Answer from the drawing. Dimensions are ordinates in mm from the lowest x, y and z of the part. A direction names the side the tool comes from. Round coordinates to 2 decimals unless told otherwise and drop trailing zeros. Write each loop counter-clockwise with the first axis right and the second up, starting at its lowest first coordinate (ties: lowest second). Pieces come first, ordered by that corner, then holes.
1. Find section A-A (y = 14.92). Write down the section's boundary in (x, z).
2. Flat-ended cylindrical pins translate along their axes: pin 1 Ø5 at (y, z) = (11.5, 9) entering from -X; pin 2 Ø1.5 at (x, z) = (1, 1.5) entering from -Y; pin 3 Ø1.5 at (x, z) = (1, 1) entering from +Y; pin 4 Ø1.5 at (x, y) = (1, 12.5) entering from -Z. Find the tip coordinate at first contact, or state that the pin passes through.
3. A tool of negligible diameter and unlimited length cuts with its end or side. For the marked faces 5, 6, 7, 8 and 9, from which of +Z, -Z, +X, -X, +Y, -Y can it reach the whole face along a straight path? Write none if from no direction.
4. Find section C-C (x = 0.75). Write down the section's boundary in (y, z), and give its area (3 significant figures).
5. Find section B-B (z = 5.91). Write down the section's boundary in (x, y).
6. Find section D-D (z = 1.5). Write down the section's boundary in (x, y).
7. Straight lines are drawn through the part: probe 1 along Y at (x, z) = (1.9, 5.91); probe 2 along Z at (x, y) = (0.6, 5); probe 3 along Y at (x, z) = (1.95, 7). For each, find the intervals that lie inside material, in ascending order.
8. Determine the mould class of the marked faces 1, 2, 3 and 4 for opening direction Z: pulls with the +Z half, pulls with the -Z half, needs draft (parallel to the pull), parting line crosses it, or undercut.
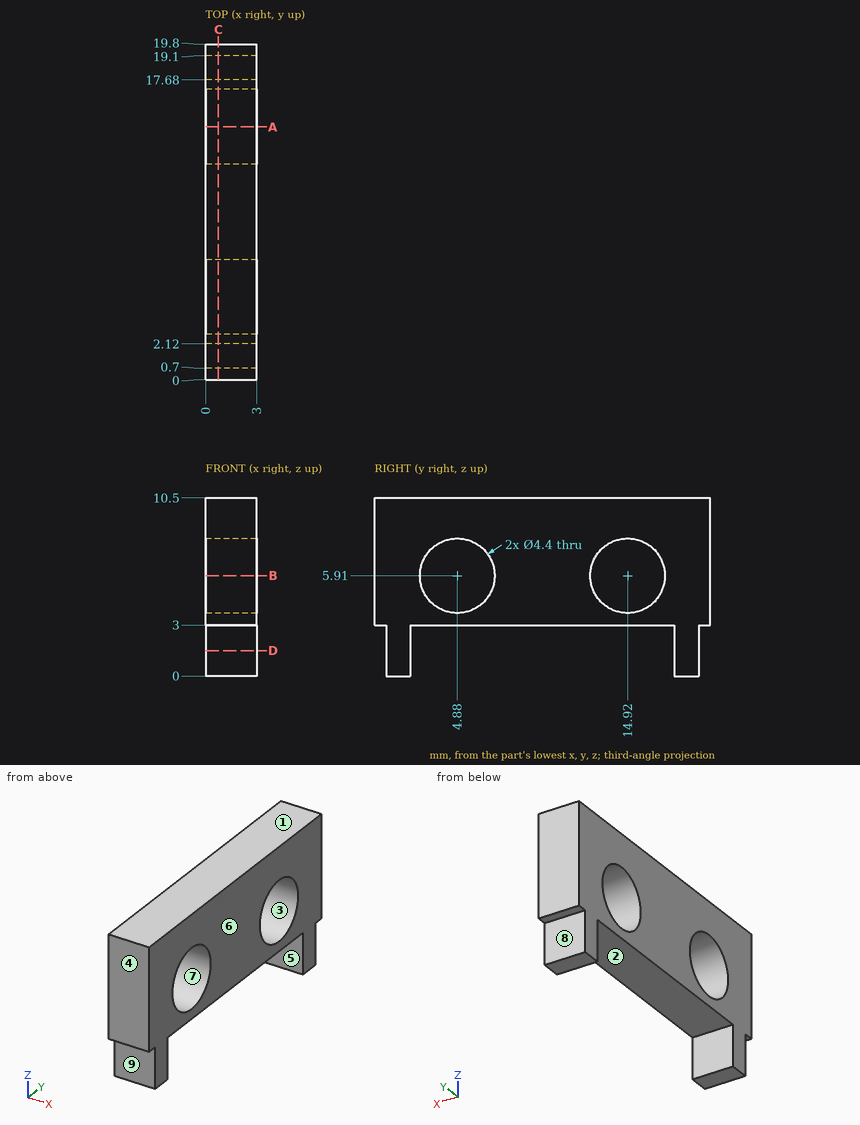
Worked answers:
1. outline: (0, 3) - (3, 3) - (3, 3.71) - (0, 3.71) - close; (0, 8.11) - (3, 8.11) - (3, 10.5) - (0, 10.5) - close
2. pin 1: stops at x = 0
2. pin 2: stops at y = 0.7
2. pin 3: stops at y = 19.1
2. pin 4: stops at z = 3
3. face 5: -Z, +X, -X
3. face 6: +Z, -Z, +X, +Y, -Y
3. face 7: +X, -X
3. face 8: -Z, +X, -X, +Y
3. face 9: -Z, +X, -X, -Y
4. outline: (0, 3) - (0.7, 3) - (0.7, 0) - (2.12, 0) - (2.12, 3) - (17.68, 3) - (17.68, 0) - (19.1, 0) - (19.1, 3) - (19.8, 3) - (19.8, 10.5) - (0, 10.5) - close; hole circle Ø4.4 at (4.88, 5.91); hole circle Ø4.4 at (14.92, 5.91)
4. area: 127 mm2
5. outline: (0, 0) - (3, 0) - (3, 2.68) - (0, 2.68) - close; (0, 7.08) - (3, 7.08) - (3, 12.72) - (0, 12.72) - close; (0, 17.12) - (3, 17.12) - (3, 19.8) - (0, 19.8) - close
6. outline: (0, 0.7) - (3, 0.7) - (3, 2.12) - (0, 2.12) - close; (0, 17.68) - (3, 17.68) - (3, 19.1) - (0, 19.1) - close
7. probe 1: y = 0 to 2.68, 7.08 to 12.72, 17.12 to 19.8
7. probe 2: z = 3 to 3.71, 8.11 to 10.5
7. probe 3: y = 0 to 2.97, 6.79 to 13.01, 16.83 to 19.8
8. face 1: pulls with the +Z half
8. face 2: pulls with the -Z half
8. face 3: undercut
8. face 4: needs draft
